```python
from build123d import *

# Parameters (mm, degrees)
F0_R      = 42.35
F1_DEPTH  = 26
F2_R      = 35
F3_DEPTH  = 12
F6_W      = 23
F6_H      = 100
F7_DEPTH  = 12
F8_R      = 2.6
F9_DEPTH  = 2
F12_R     = 5
F13_DEPTH = 26.001


with BuildPart() as f1:
    # F0 (on Top) → F1 (new body)
    with BuildSketch(Plane.XY):
        Circle(F0_R)
    extrude(amount=F1_DEPTH)

    # F2 (on face) → F3 (cut)
    with BuildSketch(Plane.XY.offset(26)):
        Circle(F2_R)
    extrude(amount=-F3_DEPTH, mode=Mode.SUBTRACT)

    # F6 (on face) → F7 (cut)
    with BuildSketch(Plane.XY.offset(26)):
        Rectangle(F6_W, F6_H)
    extrude(amount=-F7_DEPTH, mode=Mode.SUBTRACT)

    # F8 (on face) → F9 (cut)
    with BuildSketch(Plane.XY.offset(14)):
        with Locations((-20.152543, 20.152543)):
            Circle(F8_R)
        with Locations((20.152543, 20.152543)):
            Circle(F8_R)
        with Locations((20.152543, -20.152543)):
            Circle(F8_R)
        with Locations((-20.152543, -20.152543)):
            Circle(F8_R)
    extrude(amount=-F9_DEPTH, mode=Mode.SUBTRACT)

    # F10 (on Front) → F11 (revolve)
    with BuildSketch(Plane.XZ):
        Polygon((22.075, 20.8), (0, 20.8), (0, 14), (22.975, 14), (22.975, 15.9), align=None)
    revolve(axis=Axis((0, 0, 8.84423), (0, 0, 1)))

    # F12 (on face) → F13 (cut, through all)
    with BuildSketch(Plane(origin=(0, 0, 0), x_dir=(1, 0, 0), z_dir=(0, 0, -1))):
        Circle(F12_R)
    extrude(amount=-F13_DEPTH, mode=Mode.SUBTRACT)


solid = f1.part
```
Check sheet for the modelled part. Datum: model origin and axes. Units: mm. A direction names the side the tool comes from. Round coordinates to 2 decimals unless told otherwise and drop trailing zeros. Write each loop counter-clockwise with the first axis right and the second up, starting at its lowest first coordinate (ties: lowest second). Pieces come first, ordered by that corner, then holes. Notation, with made-up numbers: (10.5, 39) -> (23.5, 39) arc R16 cw to (23.5, 65) -> close; hole circle Ø9 at (44, 2). An arc over 180 degrees is marked (long way). One line per question, with ' | ' between items. Start each with the question number.
1. Depth check by flat-ended pin: pin 1 (4 mm diameter, centred on x = 21, y = -20, fed in from +Z); pin 2 (4 mm diameter, centred on y = -36.5, z = 20, fed in from -X); pin 3 (1.5 mm diameter, centred on x = -9.5, z = 11.5, fed in from +Y). Enter the tip coordinate at first touch or a pass-through.
2. Sectioned sample at B-B, the plane z = 24.25. Record the cut outline in (x, y).
3. Sectioned sample at A-A, the plane x = 0. Record the cut outline in (y, z) (3 decimals).
4. Scan lines: line 1 along X through (y, z) = (0, 10); line 2 along X through (y, z) = (-10.5, 15.75); line 3 along X through (y, z) = (17, 15.5). Record each from-to range of solid material in increasing order. Write a range as from..to.
5. Sectioned sample at D-D, the plane z = 4.5. Record the cut outline in (x, y), then the cut area to 3 significant figures.
6. Release check for a two-part mould opening along X. For faces 1 (the face through (36, 6, 26)), 2 (the face through (40.4, 12.7, 12.8)), 3 (the face through (-20, 20, 12)) record: +X half, -X half, draft (parallel to the pull), parting line (faces both ways), or undercut.
7. Sectioned sample at C-C, the plane y = 0. Record the cut outline in (x, z) (3 decimals).
8. Set-up check for faces 4 (the face through (-11.5, 37, 20)), 5 (the face through (11.5, -37, 20)), 6 (the face through (-1, -9, 0)), 7 (the face through (-20, -20, 12)): record each of +Z, -Z, +X, -X, +Y, -Y from which the full face is reachable in a straight line by a thin tool's end or side.
Taken from the geometry:
1) pin 1: stops at z = 14 | pin 2: stops at x = -24.56 | pin 3: stops at y = 41.44
2) outline: (-11.5, -40.76) -> (-11.5, -33.06) arc R35 cw to (-11.5, 33.06) -> (-11.5, 40.76) arc R42.35 ccw to start; (11.5, -40.76) arc R42.35 ccw to (11.5, 40.76) -> (11.5, 33.06) arc R35 cw to (11.5, -33.06) -> close
3) outline: (-42.35, 0) -> (-5, 0) -> (-5, 20.8) -> (-22.075, 20.8) -> (-22.975, 15.9) -> (-22.975, 14) -> (-42.35, 14) -> close; (5, 0) -> (42.35, 0) -> (42.35, 14) -> (22.975, 14) -> (22.975, 15.9) -> (22.075, 20.8) -> (5, 20.8) -> close
4) line 1: x = -42.35..-5, 5..42.35 | line 2: x = -41.03..-33.39, -20.44..20.44, 33.39..41.03 | line 3: x = -38.79..-30.59, -15.45..15.45, 30.59..38.79
5) outline: circle Ø84.7 at (0, 0); hole circle Ø10 at (0, 0) | area: 5,560 mm^2
6) face 1: draft | face 2: parting line | face 3: undercut
7) outline: (-42.35, 0) -> (-5, 0) -> (-5, 20.8) -> (-22.075, 20.8) -> (-22.975, 15.9) -> (-22.975, 14) -> (-35, 14) -> (-35, 26) -> (-42.35, 26) -> close; (5, 0) -> (42.35, 0) -> (42.35, 26) -> (35, 26) -> (35, 14) -> (22.975, 14) -> (22.975, 15.9) -> (22.075, 20.8) -> (5, 20.8) -> close
8) face 4: +Z, +Y | face 5: +Z, -Y | face 6: -Z, +X, -X, +Y, -Y | face 7: +Z
